Input: part model. Units: mm. Frame: model coordinates. Face numbers are marked on the shaded views. Coordinates: 2 decimals unless noted, no trailing zeros. Loops run counter-clockwise (first coordinate to the right, second up) from the corner with the lowest first, then second, coordinate; pieces in that order, holes last.
(1) Contact query for flat-ended pins moving along their axis: P1, Ø5, axis at y = 2.5, z = 27, coming from the -X side; P2, Ø1.5, axis at x = 11, y = 3.5, coming from the -Z side; P3, Ø5, axis at y = 6.5, z = -19, coming from the +X side. Output: stop coordinate, or through.
(2) Section D-D, the plane x = 51. Return loops of the section in (y, z).
(3) Mould query, pull axis Y, two halves, no side actions, for the marked faces 1, 2 and 3. Classes: released by +Y, released by -Y, zero draft, split by the parting line, or undercut.
(4) Section B-B, the plane z = 0. Return loops of the section in (x, y).
(5) Line query: L1, parallel to X at y = 4.5, z = 17; L2, parallel to X at y = 3.75, z = 26.5; L3, parallel to Z at x = -50, y = 6.75. Output: solid intervals per line, ascending.
(6) Section C-C, the plane z = 51. Return loops of the section in (x, y), then the cut area to 3 significant figures.
(7) Section A-A, the plane x = 0. Return loops of the section in (y, z).
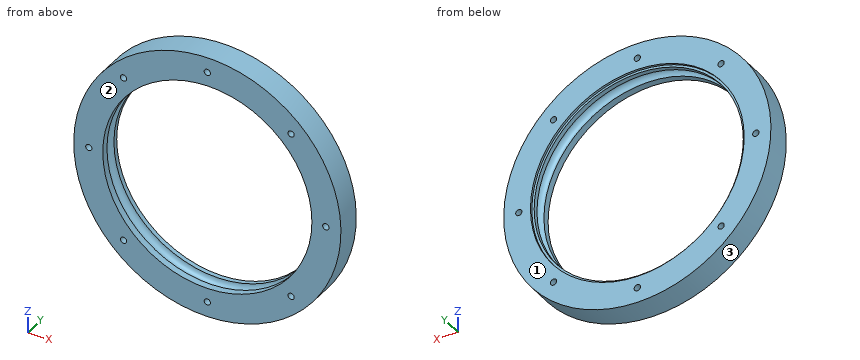
```python
from build123d import *

# Parameters (mm, degrees)
SKETCH2_W          = 11.5
SKETCH2_H          = 1
SKETCH3_R          = 1.35
CUT_EXTRUDE1_DEPTH = 83.057906383


with BuildPart() as part:
    # Sketch2 → Revolve1 (revolve)
    with BuildSketch(Plane.XY, mode=Mode.PRIVATE) as revolve1_sk:
        with Locations((-51.75, 10.5)):
            Rectangle(SKETCH2_W, SKETCH2_H)
        with BuildLine():
            Line((-45, 8), (-45, 10))
            Line((-45, 10), (-46, 10))
            Line((-46, 10), (-57.5, 10))
            Line((-57.5, 10), (-57.5, 0))
            Line((-57.5, 0), (-45, 0))
            Line((-45, 0), (-45, 3))
            ThreePointArc((-45, 3), (-47.5, 5.5), (-45, 8))
        make_face()
    revolve(revolve1_sk.sketch.rotate(Axis((0, 0, 0), (0, 1, 0)), 270), axis=Axis((0, 0, 0), (0, 1, 0)))

    # Sketch3 → Cut-Extrude1 (cut, through all)
    with BuildSketch(Plane(origin=(0, 11, 0), x_dir=(1, 0, 0), z_dir=(0, 1, 0))):
        with Locations(Location((-36.062445841, -36.062445841, 0), (0, 0, 270))):
            Circle(SKETCH3_R)
        with Locations(Location((0, -51, 0), (0, 0, 270))):
            Circle(SKETCH3_R)
        with Locations(Location((36.062445841, -36.062445841, 0), (0, 0, 270))):
            Circle(SKETCH3_R)
        with Locations(Location((51, 0, 0), (0, 0, 270))):
            Circle(SKETCH3_R)
        with Locations(Location((36.062445841, 36.062445841, 0), (0, 0, 270))):
            Circle(SKETCH3_R)
        with Locations(Location((0, 51, 0), (0, 0, 270))):
            Circle(SKETCH3_R)
        with Locations(Location((-36.062445841, 36.062445841, 0), (0, 0, 270))):
            Circle(SKETCH3_R)
        with Locations(Location((-51, 0, 0), (0, 0, 270))):
            Circle(SKETCH3_R)
    extrude(amount=-CUT_EXTRUDE1_DEPTH, mode=Mode.SUBTRACT)


solid = part.part
```
Report:
1. P1: stops at x = -52.02
1. P2: stops at z = -56.58
1. P3: stops at x = 55.08
2. outline: (0, -26.56) - (11, -26.56) - (11, -1.35) - (0, -1.35) - close; (0, 1.35) - (11, 1.35) - (11, 26.56) - (0, 26.56) - close
3. face 1: released by +Y
3. face 2: released by -Y
3. face 3: zero draft
4. outline: (-57.5, 0) - (-52.35, 0) - (-52.35, 11) - (-57.5, 11) - close; (-49.65, 0) - (-45, 0) - (-45, 3) arc R2.5 cw to (-45, 8) - (-45, 10) - (-46, 10) - (-46, 11) - (-49.65, 11) - close; (45, 0) - (49.65, 0) - (49.65, 11) - (46, 11) - (46, 10) - (45, 10) - (45, 8) arc R2.5 cw to (45, 3) - close; (52.35, 0) - (57.5, 0) - (57.5, 11) - (52.35, 11) - close
5. L1: x = -54.93 to -44.13, 44.13 to 54.93
5. L2: x = -51.03 to -38.56, 38.56 to 51.03
5. L3: z = -28.39 to -0.91, 0.91 to 28.39
6. outline: (-26.56, 0) - (-1.35, 0) - (-1.35, 11) - (-26.56, 11) - close; (1.35, 0) - (26.56, 0) - (26.56, 11) - (1.35, 11) - close
6. area: 555 mm2
7. outline: (0, -57.5) - (11, -57.5) - (11, -52.35) - (0, -52.35) - close; (0, -49.65) - (11, -49.65) - (11, -46) - (10, -46) - (10, -45) - (8, -45) arc R2.5 cw to (3, -45) - (0, -45) - close; (0, 45) - (3, 45) arc R2.5 cw to (8, 45) - (10, 45) - (10, 46) - (11, 46) - (11, 49.65) - (0, 49.65) - close; (0, 52.35) - (11, 52.35) - (11, 57.5) - (0, 57.5) - close
